Geometry check sheet. Reference: the model listing, model coordinates, mm. A direction names the side the tool comes from. Give positions to 0.01 mm unless a question says otherwise; leave off trailing zeros. Write each loop counter-clockwise with the first axis right and the second up, starting at its lowest first coordinate (ties: lowest second). Pieces come first, ordered by that corner, then holes.
(1) Depth check by flat-ended pin: P1, Ø1.5, axis at y = -1.5, z = 54.5, coming from the +X side; P2, Ø5, axis at x = -0.5, z = 60.5, coming from the -Y side; P3, Ø1, axis at x = 5.5, z = 60.5, coming from the +Y side. Enter the tip coordinate at first touch or a pass-through.
(2) Cross-section at A-A (z = 6.5). Record the boundary of the cut face in (x, y), and give its area (3 significant figures).
(3) Cross-section at C-C (z = 27). Record the boundary of the cut face in (x, y).
(4) Cross-section at B-B (z = 36). Record the boundary of the cut face in (x, y).
(5) Tool access check on faces 1 (the flat face through (-3, -6, 25.4)), 2 (the flat face through (3, -6, 25.4)), 3 (the flat face through (7, 0, 25.4)). Record the directions out of +Z, -Z, +X, -X, +Y, -Y that give a thin tool (end or side, any length) a straight path to the whole face; none if there is none.
(6) Thickness scan on line 1 along Y through (x, z) = (0, 62.5); line 2 along X through (y, z) = (0, 16); line 3 along X through (y, z) = (0, 53). Record the ranges inside material, lowest first.
Autodesk Inventor part; units mm, degrees
ref_plane "Work Plane1" through (0, 0, 33.3375) normal (0, 0, 1) x (1, 0, 0)
ref_plane "YZ Plane" through (0, 0, 0) normal (1, 0, 0) x (0, 1, 0)
ref_plane "XZ Plane" through (0, 0, 0) normal (0, 1, 0) x (-1, 0, 0)
sketch "Sketch1" plane through (0, 0, 0) normal (0, 0, 1) x (1, 0, 0)
  line L0 (-7.3323, 0) -> (-3.6662, 6.35)
  line L1 (-3.6662, 6.35) -> (3.6662, 6.35)
  line L2 (3.6662, 6.35) -> (7.3323, 0)
  line L3 (7.3323, 0) -> (3.6662, -6.35)
  line L4 (3.6662, -6.35) -> (-3.6662, -6.35)
  line L5 (-3.6662, -6.35) -> (-7.3323, 0)
  point P0 (0, 0)
  point P1 (0, 0)
  dimension "d0" = 12.7
extrude "Extrusion1" add sketch "Sketch1" along normal blind 25.4
sketch "Sketch2" plane through (0, 0, 25.4) normal (0, 0, 1) x (1, 0, 0)
  circle A0 centre (0, 0) radius 6.35
  circle A1 centre (0, 0) radius 7.9375
  dimension "d3" = 12.7
  dimension "d18" = 15.875
extrude "Extrusion2" add sketch "Sketch2" along normal blind 7.9375 contours A0
ref_plane "Work Plane1" through (0, 0, 33.3375) normal (0, 0, 1) x (1, 0, 0)
sketch "Sketch3" plane through (0, 0, 33.3375) normal (0, 0, 1) x (1, 0, 0)
  circle A0 centre (0, 0) radius 6.35
  line L0 (-6.4158, 0) -> (-3.2079, 5.5562)
  line L1 (-3.2079, 5.5562) -> (3.2079, 5.5563)
  line L2 (3.2079, 5.5563) -> (6.4158, 0)
  line L3 (6.4158, 0) -> (3.2079, -5.5563)
  line L4 (3.2079, -5.5563) -> (-3.2079, -5.5563)
  line L5 (-3.2079, -5.5563) -> (-6.4158, 0)
  dimension "d7" = 11.1125
extrude "Extrusion3" add sketch "Sketch3" along normal blind 44.45 contours A0 L3 L4 L5 L0 L1 L2 | A0 L2 L3 | A0 L1 L2 | L3 L4 A0 | A0 L0 L1 | L4 L5 A0 | A0 L5 L0
extrude "Extrusion6" cut sketch "Sketch2" along normal through all
fillet "Fillet1" radius 0.508 6 edges at (0, 5.5562, 33.3375) (4.8119, 2.7781, 33.3375) (4.8119, -2.7781, 33.3375) (0, -5.5563, 33.3375) (-4.8119, -2.7781, 33.3375) (-4.8119, 2.7781, 33.3375)
sketch "Sketch6" plane through (0, 0, 77.7875) normal (0, 0, 1) x (1, 0, 0)
  arc A0 (-3.0742, 5.5562) -> (-3.2748, 5.4404) centre (0, 0) ccw
hole "Hole2" at (0, 0, 77.7875) direction (0, 0, -1) diameter 6.5278 end through all
properties part number "Base OutputShaft"
Reply:
1. P1: stops at x = 5.98
1. P2: stops at y = -5.56
1. P3: stops at y = 2.45
2. outline: (-7.33, 0) - (-3.67, -6.35) - (3.67, -6.35) - (7.33, 0) - (3.67, 6.35) - (-3.67, 6.35) - close; hole circle Ø6.53 at (0, 0)
2. area: 106 mm2
3. outline: circle Ø12.7 at (0, 0); hole circle Ø6.53 at (0, 0)
4. outline: (-6.35, -0.12) - (-3.27, -5.44) arc R6.35 ccw to (-3.07, -5.56) - (3.07, -5.56) arc R6.35 ccw to (3.27, -5.44) - (6.35, -0.12) arc R6.35 ccw to (6.35, 0.12) - (3.27, 5.44) arc R6.35 ccw to (3.07, 5.56) - (-3.07, 5.56) arc R6.35 ccw to (-3.27, 5.44) - (-6.35, 0.12) arc R6.35 ccw to start; hole circle Ø6.53 at (0, 0)
5. face 1: +Z, -X, -Y
5. face 2: +Z, +X, -Y
5. face 3: +Z, +X
6. line 1: y = -5.56 to -3.26, 3.26 to 5.56
6. line 2: x = -7.33 to -3.26, 3.26 to 7.33
6. line 3: x = -6.35 to -3.26, 3.26 to 6.35
